from build123d import *

# Parameters (mm, degrees)
F0_R     = 4
F1_DEPTH = 4
F2_DEPTH = 4
F3_DEPTH = 25
F4_R     = 2
F5_R     = 0.5


with BuildPart() as f1:
    # F0 (on Top) → F1 (new body)
    with BuildSketch(Plane.XY):
        with BuildLine():
            ThreePointArc((4.1287042683, -5.02033874), (5.8773539005, -2.776096383), (6.5, 0))
            ThreePointArc((6.5, 0), (6.4779859765, 0.534506958), (6.412093019, 1.0653934086))
            ThreePointArc((6.412093019, 1.0653934086), (5.020338785, 4.1287042137), (2.2833888805, 6.0857321023))
            ThreePointArc((2.2833888805, 6.0857321023), (-1.0653932869, 6.4120930393), (-4.1287041813, 5.0203388116))
            ThreePointArc((-4.1287041813, 5.0203388116), (-6.0857321431, 2.2833887717), (-6.4120930076, -1.0653934773))
            ThreePointArc((-6.4120930076, -1.0653934773), (-5.020338751, -4.1287042549), (-2.2833888456, -6.0857321153))
            ThreePointArc((-2.2833888456, -6.0857321153), (1.0653933609, -6.412093027), (4.1287042683, -5.02033874))
        make_face()
        Circle(F0_R, mode=Mode.SUBTRACT)
        with BuildLine():
            ThreePointArc((6.412093019, 1.0653934086), (6.4779859765, 0.534506958), (6.5, 0))
            ThreePointArc((6.5, 0), (5.8773539005, -2.776096383), (4.1287042683, -5.02033874))
            Line((4.1287042683, -5.02033874), (7.027198158, -2.6366303082))
            Line((7.027198158, -2.6366303082), (6.412093019, 1.0653934086))
        make_face()
        with BuildLine():
            ThreePointArc((2.2833888805, 6.0857321023), (5.020338785, 4.1287042137), (6.412093019, 1.0653934086))
            Line((6.412093019, 1.0653934086), (5.7969879062, 4.7674169681))
            Line((5.7969879062, 4.7674169681), (2.2833888805, 6.0857321023))
        make_face()
        with BuildLine():
            Line((1.2302102517, -7.4040472763), (4.1287042683, -5.02033874))
            ThreePointArc((4.1287042683, -5.02033874), (1.0653933609, -6.412093027), (-2.2833888456, -6.0857321153))
            Line((-2.2833888456, -6.0857321153), (1.2302102517, -7.4040472763))
        make_face()
        with BuildLine():
            ThreePointArc((-4.1287041813, 5.0203388116), (-1.0653932869, 6.4120930393), (2.2833888805, 6.0857321023))
            Line((2.2833888805, 6.0857321023), (-1.2302102517, 7.4040472763))
            Line((-1.2302102517, 7.4040472763), (-4.1287041813, 5.0203388116))
        make_face()
        with BuildLine():
            Line((-5.7969879062, -4.7674169681), (-2.2833888456, -6.0857321153))
            ThreePointArc((-2.2833888456, -6.0857321153), (-5.020338751, -4.1287042549), (-6.4120930076, -1.0653934773))
            Line((-6.4120930076, -1.0653934773), (-5.7969879062, -4.7674169681))
        make_face()
        with BuildLine():
            ThreePointArc((-6.4120930076, -1.0653934773), (-6.0857321431, 2.2833887717), (-4.1287041813, 5.0203388116))
            Line((-4.1287041813, 5.0203388116), (-7.027198158, 2.6366303082))
            Line((-7.027198158, 2.6366303082), (-6.4120930076, -1.0653934773))
        make_face()
        Circle(F0_R)
        Polygon((-2.6272431226, -2.2577851038), (-3.2689208174, 1.1463667342), (-0.6416776948, 3.404151838), (2.6272431226, 2.2577851038), (3.2689208174, -1.1463667342), (0.6416776948, -3.404151838), align=None, mode=Mode.SUBTRACT)
        Polygon((-0.6416776948, 3.404151838), (-3.2689208174, 1.1463667342), (-2.6272431226, -2.2577851038), (0.6416776948, -3.404151838), (3.2689208174, -1.1463667342), (2.6272431226, 2.2577851038), align=None)
    extrude(amount=-F1_DEPTH)

    # F0 (on Top) → F2 (join)
    with BuildSketch(Plane.XY):
        with BuildLine():
            ThreePointArc((4.1287042683, -5.02033874), (5.8773539005, -2.776096383), (6.5, 0))
            ThreePointArc((6.5, 0), (6.4779859765, 0.534506958), (6.412093019, 1.0653934086))
            ThreePointArc((6.412093019, 1.0653934086), (5.020338785, 4.1287042137), (2.2833888805, 6.0857321023))
            ThreePointArc((2.2833888805, 6.0857321023), (-1.0653932869, 6.4120930393), (-4.1287041813, 5.0203388116))
            ThreePointArc((-4.1287041813, 5.0203388116), (-6.0857321431, 2.2833887717), (-6.4120930076, -1.0653934773))
            ThreePointArc((-6.4120930076, -1.0653934773), (-5.020338751, -4.1287042549), (-2.2833888456, -6.0857321153))
            ThreePointArc((-2.2833888456, -6.0857321153), (1.0653933609, -6.412093027), (4.1287042683, -5.02033874))
        make_face()
        Circle(F0_R, mode=Mode.SUBTRACT)
        Circle(F0_R)
        Polygon((-2.6272431226, -2.2577851038), (-3.2689208174, 1.1463667342), (-0.6416776948, 3.404151838), (2.6272431226, 2.2577851038), (3.2689208174, -1.1463667342), (0.6416776948, -3.404151838), align=None, mode=Mode.SUBTRACT)
        with BuildLine():
            ThreePointArc((-4.1287041813, 5.0203388116), (-1.0653932869, 6.4120930393), (2.2833888805, 6.0857321023))
            Line((2.2833888805, 6.0857321023), (-1.2302102517, 7.4040472763))
            Line((-1.2302102517, 7.4040472763), (-4.1287041813, 5.0203388116))
        make_face()
        with BuildLine():
            ThreePointArc((-6.4120930076, -1.0653934773), (-6.0857321431, 2.2833887717), (-4.1287041813, 5.0203388116))
            Line((-4.1287041813, 5.0203388116), (-7.027198158, 2.6366303082))
            Line((-7.027198158, 2.6366303082), (-6.4120930076, -1.0653934773))
        make_face()
        with BuildLine():
            Line((-5.7969879062, -4.7674169681), (-2.2833888456, -6.0857321153))
            ThreePointArc((-2.2833888456, -6.0857321153), (-5.020338751, -4.1287042549), (-6.4120930076, -1.0653934773))
            Line((-6.4120930076, -1.0653934773), (-5.7969879062, -4.7674169681))
        make_face()
        with BuildLine():
            ThreePointArc((2.2833888805, 6.0857321023), (5.020338785, 4.1287042137), (6.412093019, 1.0653934086))
            Line((6.412093019, 1.0653934086), (5.7969879062, 4.7674169681))
            Line((5.7969879062, 4.7674169681), (2.2833888805, 6.0857321023))
        make_face()
        with BuildLine():
            ThreePointArc((6.412093019, 1.0653934086), (6.4779859765, 0.534506958), (6.5, 0))
            ThreePointArc((6.5, 0), (5.8773539005, -2.776096383), (4.1287042683, -5.02033874))
            Line((4.1287042683, -5.02033874), (7.027198158, -2.6366303082))
            Line((7.027198158, -2.6366303082), (6.412093019, 1.0653934086))
        make_face()
        with BuildLine():
            Line((1.2302102517, -7.4040472763), (4.1287042683, -5.02033874))
            ThreePointArc((4.1287042683, -5.02033874), (1.0653933609, -6.412093027), (-2.2833888456, -6.0857321153))
            Line((-2.2833888456, -6.0857321153), (1.2302102517, -7.4040472763))
        make_face()
    extrude(amount=F2_DEPTH)

    # F0 (on Top) → F3 (join)
    with BuildSketch(Plane.XY):
        Circle(F0_R)
        Polygon((-2.6272431226, -2.2577851038), (-3.2689208174, 1.1463667342), (-0.6416776948, 3.404151838), (2.6272431226, 2.2577851038), (3.2689208174, -1.1463667342), (0.6416776948, -3.404151838), align=None, mode=Mode.SUBTRACT)
        Polygon((-0.6416776948, 3.404151838), (-3.2689208174, 1.1463667342), (-2.6272431226, -2.2577851038), (0.6416776948, -3.404151838), (3.2689208174, -1.1463667342), (2.6272431226, 2.2577851038), align=None)
    extrude(amount=-F3_DEPTH)

    # F4
    f4_edges = [f1.edges().sort_by_distance(p)[0] for p in [
        (-4, 0, -25),
    ]]
    fillet(f4_edges, radius=F4_R)

    # F5
    f5_edges = [f1.edges().sort_by_distance(p)[0] for p in [
        (-6.412093, -1.065393, 4),
        (-2.283389, -6.085732, 4),
        (4.128704, -5.020339, 4),
        (6.412093, 1.065393, 4),
        (2.283389, 6.085732, 4),
        (-4.128704, 5.020339, 4),
    ]]
    fillet(f5_edges, radius=F5_R)


solid = f1.part
Here's how the part is built. I have some questions about the finished solid (model axes, mm). A direction names the side the tool comes from. Coordinates: 2 decimals unless noted, no trailing zeros. Write each loop counter-clockwise with the first axis right and the second up, starting at its lowest first coordinate (ties: lowest second). Pieces come first, ordered by that corner, then holes.
Item 1: On a 3-axis mill with a long thin cutter (end or side, diameter ignored), from which of +Z, -Z, +X, -X, +Y, -Y can I reach the whole of each face in a straight line? I mean faces 1 (the flat face through (3, 2, 4)), 2 (the flat face through (3, -3, -4)), 3 (the flat face through (1.97, -2.26, 1.97)). Say none if no direction works.
Item 2: I want a section at A-A on z = 1. Write out the boundary of the cut face in (x, y).
Item 3: I want a section at B-B on z = -20.75. Write out the boundary of the cut face in (x, y), and give its area (3 significant figures).
Item 4: If I drill on line 1 (Z direction, x = -1.5, y = -1); line 2 (Z direction, x = -4.5, y = 3); line 3 (Y direction, x = 0, z = 1), over which ranges is the centre line in solid material (lowest first)?
Item 5: Will these pins go through, and if not, where does the flat tip stop? pin 1 (2 mm diameter, centred on x = -1.5, y = -1, fed in from +Z); pin 2 (8 mm diameter, centred on x = -2.5, z = -21.5, fed in from +Y); pin 3 (5 mm diameter, centred on x = -4, y = -3.5, fed in from -Z).
Item 6: If we mould it in two halves opening along X, with no side actions, what happens to faces 4 (the flat face through (0, 0, 0)), 5 (the cylindrical face through (-0.867, -3.905, -13.367)), 6 (the flat face through (0, 0, -25))? For each: +X half, -X half, draft (parallel to the pull), parting line (faces both ways), or undercut.
Findings below:
1. face 1: +Z, +X, -X, +Y, -Y
1. face 2: -Z
1. face 3: +Z
2. outline: (-7.03, 2.64) - (-5.8, -4.77) - (1.23, -7.4) - (7.03, -2.64) - (5.8, 4.77) - (-1.23, 7.4) - close; hole (-3.27, 1.15) - (-2.63, -2.26) - (0.64, -3.4) - (3.27, -1.15) - (2.63, 2.26) - (-0.64, 3.4) - close
3. outline: circle Ø8 at (0, 0)
3. area: 50.3 mm2
4. line 1: z = -25 to 0
4. line 2: z = -4 to 4
4. line 3: y = -6.94 to -3.18, 3.18 to 6.94
5. pin 1: stops at z = 0
5. pin 2: stops at y = 4
5. pin 3: stops at z = -24.83
6. face 4: undercut
6. face 5: parting line
6. face 6: draft
